The model under review builds one solid part; all positions refer to its coordinate system, in mm. A direction names the side the tool comes from. Give positions to 0.01 mm unless a question says otherwise; leave off trailing zeros. Write each loop counter-clockwise with the first axis right and the second up, starting at its lowest first coordinate (ties: lowest second). Pieces come first, ordered by that corner, then holes. Notation, with made-up numbers: M 5,30.25 L 13,30.25 A29 cw 13,54.25 Z; hole C 45.5,50 d9. An arc over 180 degrees is marked long. Write each question's results on one line, items separated by ' | '. Start each with the question number.
from build123d import *

# Parameters (mm, degrees)
BOSS_EXTRUDE1_DEPTH = 6.35
FILLET1_R           = 10
SKETCH3_W           = 4
SKETCH3_H           = 6
BOSS_EXTRUDE2_DEPTH = 6.35
FILLET2_R           = 10
SKETCH4_W           = 5.85
SKETCH4_H           = 3.5
CUT_EXTRUDE1_DEPTH  = 10


with BuildPart() as part:
    # Sketch2 → Boss-Extrude1 (new body)
    with BuildSketch(Plane.XY):
        Polygon((0, -45.00147748), (0, 0), (6.35, 0), (6.35, -12.7), (75.42710801, -12.7), (75.42710801, -28.978), (6.35, -28.978), (6.35, -63.9998), (0, -63.9998), align=None)
    extrude(amount=BOSS_EXTRUDE1_DEPTH)

    # Fillet1
    fillet1_edges = [part.edges().sort_by_distance(p)[0] for p in [
        (6.35, -12.7, 3.175),
        (6.35, -28.978, 3.175),
    ]]
    fillet(fillet1_edges, radius=FILLET1_R)

    # Sketch3 → Boss-Extrude2 (add)
    with BuildSketch(Plane(origin=(0, 0, 0), x_dir=(-1, 0, 0), z_dir=(0, 0, -1))):
        with Locations((-39.89710801, -31.978)):
            Rectangle(SKETCH3_W, SKETCH3_H)
        with Locations((-55.42710801, -31.978)):
            Rectangle(SKETCH3_W, SKETCH3_H)
    extrude(amount=-BOSS_EXTRUDE2_DEPTH)

    # Fillet2
    # the kernel refuses this fillet: 10 mm, written as the material it adds along each edge
    with BuildSketch(Plane(origin=(57.42710801, -28.978, 0), x_dir=(1, 0, 0), z_dir=(0, 0, 1))) as fillet2_piece_1:
        with BuildLine():
            CenterArc((9.16515139, -10), FILLET2_R, 90, 66.421821522)
            Line((0, -6), (-0.183303028, -5.92))
            ThreePointArc((-0.183303028, -5.92), (-0.2, -3), (-0.2, 0))
            Line((-0.2, 0), (0, 0.2))
            Line((0, 0.2), (9.16515139, 0.2))
            Line((9.16515139, 0.2), (9.16515139, 0))
        make_face()
    extrude(amount=6.35)
    with BuildSketch(Plane(origin=(37.89710801, -28.978, 0), x_dir=(-1, 0, 0), z_dir=(0, 0, 1))) as fillet2_piece_2:
        with BuildLine():
            CenterArc((9.16515139, 10), FILLET2_R, 203.578178478, 66.421821522)
            Line((0, 6), (-0.183303028, 5.92))
            ThreePointArc((-0.183303028, 5.92), (-0.2, 3), (-0.2, 0))
            Line((-0.2, 0), (0, -0.2))
            Line((0, -0.2), (9.16515139, -0.2))
            Line((9.16515139, -0.2), (9.16515139, 0))
        make_face()
    extrude(amount=6.35)

    # Sketch4 → Cut-Extrude1 (cut)
    with BuildSketch(Plane(origin=(0, 0, 0), x_dir=(-1, 0, 0), z_dir=(0, 0, -1))):
        with Locations((-47.32560801, -27.228)):
            Rectangle(SKETCH4_W, SKETCH4_H)
    extrude(amount=-CUT_EXTRUDE1_DEPTH, mode=Mode.SUBTRACT)


solid = part.part
(1) Machinability: for faces 4 (the flat face through (3, -64, 3)), 5 (the flat face through (52, -28.978, 3)), 6 (the flat face through (6.35, -1, 3)), 7 (the flat face through (55, -34.978, 3)), which of the approach directions +Z, -Z, +X, -X, +Y, -Y give a long, thin tool a straight path to every point of the face, cutting with its end or side? Answer none if there is none.
(2) Wall thickness on L1, parallel to X at y = -32.5, z = 4; L2, parallel to X at y = -26.5, z = 2; L3, parallel to Y at x = 18, z = 2.5: over which ranges is each line inside the solid? List them lowest first.
(3) Add section B-B (y = -33). State the section outline as (x, z) points, then the cut area to 3 significant figures.
(4) Add section D-D (y = -58). State the section outline as (x, z) points, then the cut area to 3 significant figures.
(5) Add section A-A (z = 4.75). State the section outline as (x, y) points, then the cut area to 3 significant figures.
(6) Draft analysis for pull direction X (two halves, no side actions). For faces 1 (the flat face through (40, -34.978, 3)), 2 (the flat face through (6.35, -51, 3)), 3 (the flat face through (50.251, -27, 3)), state which applies: pulls with the +X half, pulls with the -X half, needs draft (parallel to the pull), parting line crosses it, or undercut.
(7) Add section C-C (x = 40.5). State the section outline as (y, z) points, then the cut area to 3 significant figures.
(8) Clearance check with flat-ended pins moving along their axes: P1, Ø1.9, axis at y = -55.5, z = 4.5, coming from the +X side; P2, Ø1.5, axis at y = -30.5, z = 5, coming from the +X side; P3, Ø1.2, axis at x = 56, z = 3.5, coming from the -Y side. State where each tip first meets the part, or that it passes through.
Calculated:
1) face 4: +Z, -Z, +X, -X, -Y | face 5: +Z, -Z, -Y | face 6: +Z, -Z, +X, +Y | face 7: +Z, -Z, +X, -Y
2) L1: x = 0 to 8.73, 36.35 to 41.9, 53.43 to 58.97 | L2: x = 0 to 44.4, 50.25 to 75.43 | L3: y = -28.98 to -12.7
3) outline: M 0,0 L 8.33,0 L 8.33,6.35 L 0,6.35 Z; M 36.75,0 L 41.9,0 L 41.9,6.35 L 36.75,6.35 Z; M 53.43,0 L 58.58,0 L 58.58,6.35 L 53.43,6.35 Z | area: 118 mm²
4) outline: M 0,0 L 6.35,0 L 6.35,6.35 L 0,6.35 Z | area: 40.3 mm²
5) outline: M 0,-64 L 6.35,-64 L 6.35,-38.98 A10 cw 16.35,-28.98 L 28.73,-28.98 A10 cw 37.9,-34.98 L 41.9,-34.98 L 41.9,-28.98 L 44.4,-28.98 L 44.4,-25.48 L 50.25,-25.48 L 50.25,-28.98 L 53.43,-28.98 L 53.43,-34.98 L 57.43,-34.98 A10 cw 66.59,-28.98 L 75.43,-28.98 L 75.43,-12.7 L 16.35,-12.7 A10 cw 6.35,-2.7 L 6.35,0 L 0,0 Z | area: 1,630 mm²
6) face 1: needs draft | face 2: pulls with the +X half | face 3: undercut
7) outline: M -34.98,0 L -12.7,0 L -12.7,6.35 L -34.98,6.35 Z | area: 141 mm²
8) P1: stops at x = 6.35 | P2: stops at x = 62.74 | P3: stops at y = -34.98
